Verification items for the finished model (mm, model axes). Face numbers are marked on the shaded views. Give positions to 0.01 mm unless a question says otherwise; leave off trailing zeros. Loops run counter-clockwise (first coordinate to the right, second up) from the corner with the lowest first, then second, coordinate; pieces in that order, holes last. Notation, with made-up numbers: M 78,-26.75 L 92,-26.75 A19 cw 92,-9.75 Z; hole C 45,86 d3. An arc over 180 degrees is marked long. Use a Markdown table: item, result.
from build123d import *

# Parameters (mm, degrees)
SKETCH1_W              = 20
SKETCH1_H              = 142
BOSS_EXTRUDE1_DEPTH    = 7
SKETCH2_W              = 20
SKETCH2_H              = 13
CUT_EXTRUDE1_DEPTH     = 3
LPATTERN1_COUNT        = 8
LPATTERN1_PITCH        = 17
CUT_EXTRUDE2_REACH     = 74.042
SKETCH4_W              = 6.5
SKETCH4_H              = 2
FILLET1_R              = 0.5
CHAMFER1_SIZE          = 2
LPATTERN2_COUNT        = 9
LPATTERN2_PITCH        = 17
FILLET1_OF_LPATTERN2_R = 0.5
SKETCH5_W              = 6.5
SKETCH5_H              = 15
CUT_EXTRUDE3_DEPTH     = 2
LPATTERN3_COUNT        = 8
LPATTERN3_PITCH        = 17
CUT_EXTRUDE4_REACH     = 144.524
SKETCH6_W              = 20
SKETCH6_H              = 2


with BuildPart() as part:
    # Sketch1 → Boss-Extrude1 (new body)
    with BuildSketch(Plane(origin=(0, 0, 0), x_dir=(1, 0, 0), z_dir=(0, 1, 0))):
        Rectangle(SKETCH1_W, SKETCH1_H)
    extrude(amount=BOSS_EXTRUDE1_DEPTH)

    # Sketch2 → Cut-Extrude1 (cut)
    with BuildSketch(Plane(origin=(0, 7, 0), x_dir=(1, 0, 0), z_dir=(0, 1, 0))):
        with Locations((0, 59.5)):
            Rectangle(SKETCH2_W, SKETCH2_H)
    cut_extrude1 = extrude(amount=-CUT_EXTRUDE1_DEPTH, mode=Mode.SUBTRACT)

    # LPattern1: Cut-Extrude1 ×8
    with Locations(*[(0, 0, i * LPATTERN1_PITCH) for i in range(1, LPATTERN1_COUNT)]):
        add(cut_extrude1, mode=Mode.SUBTRACT)

    # Sketch4 → Cut-Extrude2 (cut, up to next)
    with BuildSketch(Plane(origin=(0, 7, 0), x_dir=(1, 0, 0), z_dir=(0, 1, 0)), mode=Mode.PRIVATE) as cut_extrude2_sk1:
        with Locations((0, 68)):
            Rectangle(SKETCH4_W, SKETCH4_H)
    cut_extrude2_tool1 = extrude(cut_extrude2_sk1.sketch, amount=-CUT_EXTRUDE2_REACH, mode=Mode.PRIVATE) & part.part
    cut_extrude2 = cut_extrude2_tool1.solids().sort_by_distance((0, 7, -68))[0]
    add(cut_extrude2, mode=Mode.SUBTRACT)

    # Fillet1
    fillet1_edges = [part.edges().sort_by_distance(p)[0] for p in [
        (0, 7, -67),
        (0, 7, -69),
    ]]
    fillet(fillet1_edges, radius=FILLET1_R)

    # Chamfer1
    chamfer1_edges = [part.edges().sort_by_distance(p)[0] for p in [
        (-10, 7, -68.5),
        (10, 7, -68.5),
        (-10, 7, -51),
        (10, 7, 51),
        (10, 7, 34),
        (10, 7, 17),
        (10, 7, 0),
        (10, 7, -17),
        (10, 7, -34),
        (10, 7, -51),
        (-10, 7, -34),
        (-10, 7, -17),
        (-10, 7, 0),
        (-10, 7, 17),
        (-10, 7, 34),
        (-10, 7, 51),
        (-10, 7, 68.5),
        (10, 7, 68.5),
    ]]
    chamfer(chamfer1_edges, length=CHAMFER1_SIZE)

    # LPattern2: Cut-Extrude2 ×9
    with Locations(*[(0, 0, i * LPATTERN2_PITCH) for i in range(1, LPATTERN2_COUNT)]):
        add(cut_extrude2, mode=Mode.SUBTRACT)

    # Fillet1 of LPattern2
    fillet1_of_lpattern2_edges = [part.edges().sort_by_distance(p)[0] for p in [
        (0, 7, -50),
        (0, 7, -52),
        (0, 7, -33),
        (0, 7, -35),
        (0, 7, -16),
        (0, 7, -18),
        (0, 7, 1),
        (0, 7, -1),
        (0, 7, 18),
        (0, 7, 16),
        (0, 7, 35),
        (0, 7, 33),
        (0, 7, 52),
        (0, 7, 50),
        (0, 7, 69),
        (0, 7, 67),
    ]]
    fillet(fillet1_of_lpattern2_edges, radius=FILLET1_OF_LPATTERN2_R)

    # Sketch5 → Cut-Extrude3 (cut)
    with BuildSketch(Plane.XZ):
        with Locations((0, 59.5)):
            Rectangle(SKETCH5_W, SKETCH5_H)
    cut_extrude3 = extrude(amount=-CUT_EXTRUDE3_DEPTH, mode=Mode.SUBTRACT)

    # LPattern3: Cut-Extrude3 ×8
    with Locations(*[(0, 0, -i * LPATTERN3_PITCH) for i in range(1, LPATTERN3_COUNT)]):
        add(cut_extrude3, mode=Mode.SUBTRACT)

    # Cut-Extrude4: up to this face of the body (flat: up to its plane)
    cut_extrude4_end = Plane(part.part.faces().sort_by_distance((0, 3.416666667, 71))[0])
    # Sketch6 → Cut-Extrude4 (cut, up to the picked face)
    with BuildSketch(Plane(origin=(0, 0, -71), x_dir=(-1, 0, 0), z_dir=(0, 0, -1)), mode=Mode.PRIVATE) as cut_extrude4_sk1:
        with Locations((0, 6)):
            Rectangle(SKETCH6_W, SKETCH6_H)
    cut_extrude4_tool1 = split(extrude(cut_extrude4_sk1.sketch, amount=-CUT_EXTRUDE4_REACH, mode=Mode.PRIVATE), bisect_by=cut_extrude4_end, keep=Keep.BOTH, mode=Mode.PRIVATE)
    add(cut_extrude4_tool1.solids().sort_by(Axis((0, 6, -71), (0, 0, 1)))[0], mode=Mode.SUBTRACT)


solid = part.part
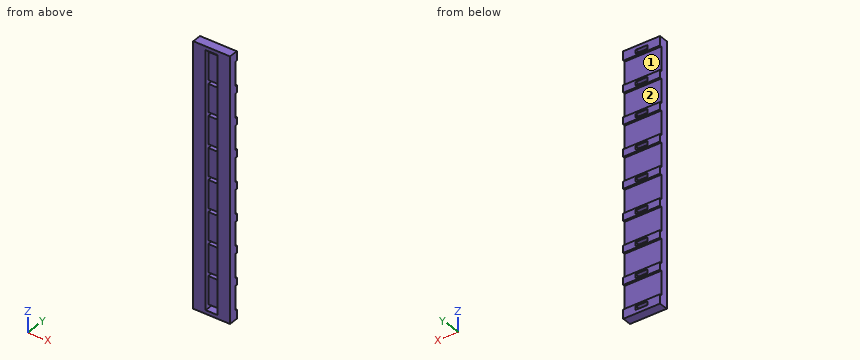
(1) Draft check along Z on the marked faces 1 and 2. Enter one of: +Z half, -Z half, draft (parallel to the pull), parting line (faces both ways), or undercut.
Results below:
| item | result |
|---|---|
| face 1 | undercut |
| face 2 | undercut |
(2) Cross-section at A-A on z = -5. Record the cut outline in (x, y).
Results below:
| item | result |
|---|---|
| outline | M -10,0 L -3.25,0 L -3.25,2 L 3.25,2 L 3.25,0 L 10,0 L 10,4 L -10,4 Z |
(3) Cross-section at B-B on y = 1.2. Record the cut outline in (x, z), then the cut area to 3 significant figures.
Results below:
| item | result |
|---|---|
| outline | M -10,-71 L 10,-71 L 10,71 L -10,71 Z; hole M -3.25,-69 L 3.25,-69 L 3.25,69 L -3.25,69 Z |
| area | 1,940 mm^2 |
(4) Gauge pin test, flat ends, axial feed: P1, Ø4, axis at x = 1, z = 37, coming from the -Y side; P2, Ø4, axis at x = 0, z = -23, coming from the +Y side; P3, Ø8, axis at x = 6, z = 13.5, coming from the -Y side. Record the tip position at first contact, or that the pin passes through.
Results below:
| item | result |
|---|---|
| P1 | y = 2 |
| P2 | y = 4 |
| P3 | y = 0 |
(5) Material ranges on line 1 (X direction, y = 4.55, z = 0); line 2 (Z direction, x = 0.75, y = 1); line 3 (Y direction, x = -0.5, z = -48.5), recorded low to high.
Results below:
| item | result |
|---|---|
| line 1 | -10 to -3.25, 3.25 to 10 |
| line 2 | -71 to -69, 69 to 71 |
| line 3 | 2 to 4 |
